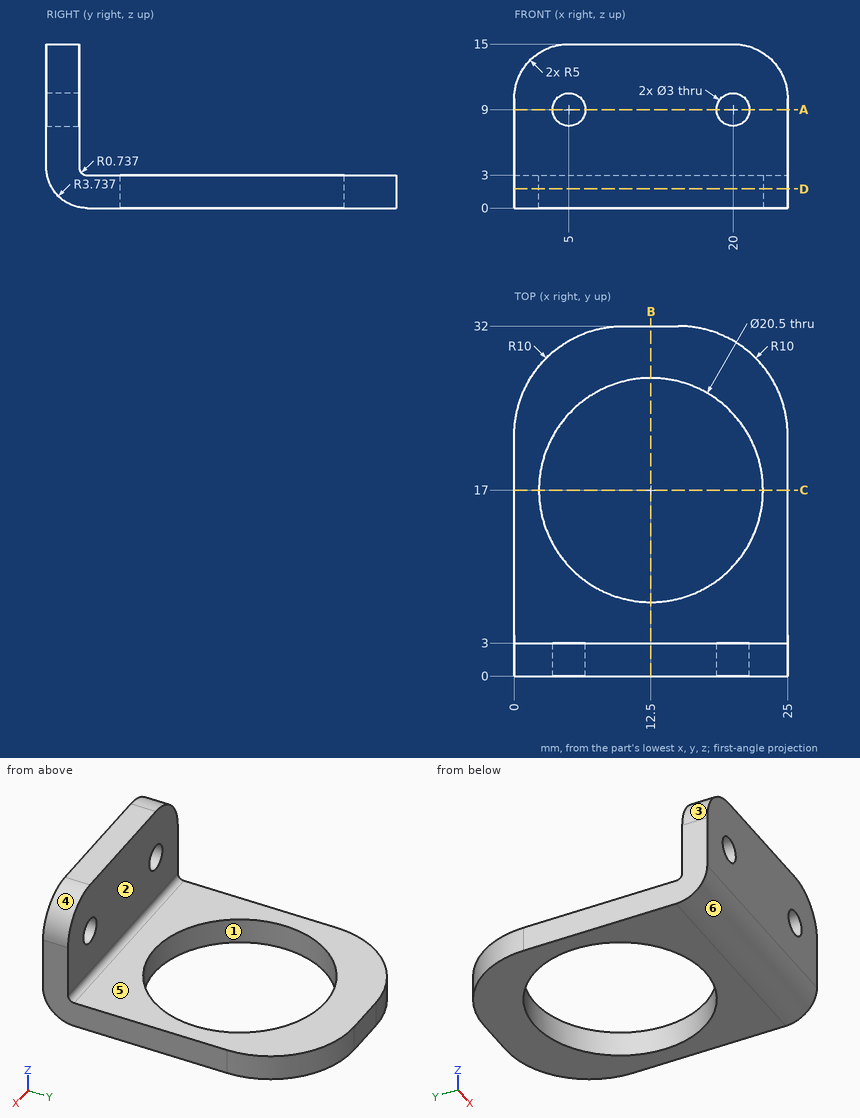
Source: three-view drawing plus pictorial views. Frame: mm from the lowest corner of the part. A direction names the side the tool comes from. Coordinates: 2 decimals unless noted, no trailing zeros. Order: outer loops, then holes, each group sorted by start corner. A loop starts at its lowest first (then second) coordinate and runs counter-clockwise, first axis right, second up.
Item 1: Pull-direction query (X, two-part tool) for the marked faces 1, 2, 3 and 4; classes: pulls with the +X half, pulls with the -X half, needs draft (parallel to the pull), parting line crosses it, or undercut.
Output values:
face 1: undercut
face 2: needs draft
face 3: pulls with the -X half
face 4: pulls with the +X half
Item 2: Cut plane B-B (x = 12.5). Return loops of the section in (y, z).
Output values:
outline: (0, 3.74) arc R3.74 ccw to (3.74, 0) - (6.75, 0) - (6.75, 3) - (3.74, 3) arc R0.74 cw to (3, 3.74) - (3, 15) - (0, 15) - close; (27.25, 0) - (32, 0) - (32, 3) - (27.25, 3) - close
Item 3: Cut plane C-C (y = 17). Return loops of the section in (x, z), plus the area to 3 significant figures.
Output values:
outline: (0, 0) - (2.25, 0) - (2.25, 3) - (0, 3) - close; (22.75, 0) - (25, 0) - (25, 3) - (22.75, 3) - close
area: 13.5 mm2
Item 4: Cut plane A-A (z = 9). Return loops of the section in (x, y).
Output values:
outline: (0, 0) - (3.5, 0) - (3.5, 3) - (0, 3) - close; (6.5, 0) - (18.5, 0) - (18.5, 3) - (6.5, 3) - close; (21.5, 0) - (25, 0) - (25, 3) - (21.5, 3) - close
Item 5: Set-up query: the marked faces 5 and 6. Return all of +Z, -Z, +X, -X, +Y, -Y with unobstructed straight access to the full face (end or side cutting, diameter ignored); none if empty.
Output values:
face 5: +Z, +X, -X, +Y
face 6: -Z, +X, -X, -Y
Item 6: Cut plane D-D (z = 1.75). Return loops of the section in (x, y).
Output values:
outline: (0, 0.57) - (25, 0.57) - (25, 22) arc R10 ccw to (15, 32) - (10, 32) arc R10 ccw to (0, 22) - close; hole circle Ø20.5 at (12.5, 17)
Item 7: Material intervals for line 1 (X direction, y = 1.4, z = 9); line 2 (Y direction, x = 12.5, z = 12.5); line 3 (Y direction, x = 12.5, z = 1.6), sorted ascending.
Output values:
line 1: x = 0 to 3.5, 6.5 to 18.5, 21.5 to 25
line 2: y = 0 to 3
line 3: y = 0.67 to 6.75, 27.25 to 32
Item 8: First-contact query: P1, Ø1.5, axis at x = 9, z = 8, coming from the +Y side; P2, Ø12.5, axis at x = 12.5, y = 17, coming from the -Z side; P3, Ø5, axis at x = 20, z = 1.5, coming from the +Y side; P4, Ø3, axis at x = 22, z = 2, coming from the -Y side. Flat tips, straight axial feed; report the tip coordinate or a pass-through.
Output values:
P1: stops at y = 3
P2: passes through
P3: stops at y = 31.68
P4: stops at y = 0.01
